```python
from build123d import *

# Parameters (mm, degrees)
SKETCH1_W               = 4
SKETCH1_H               = 2
SKETCH1_H_2             = 5
CUT_EXTRUDE1_DEPTH      = 94.386294498
CUT_EXTRUDE1_DEPTH_BACK = 94.386294498
SKETCH2_R               = 11


with BuildPart() as part:
    # Sketch1 → Revolve1 (revolve)
    with BuildSketch(Plane.YZ, mode=Mode.PRIVATE) as revolve1_sk:
        with BuildLine():
            ThreePointArc((-46, 2), (-23.174880185, 6.257119382), (0, 7.683334091))
            Line((0, 7.683334091), (0, 2))
            Line((0, 2), (-46, 2))
        make_face()
        Polygon((-46, 2), (-46, 0), (-42, 0), (0, 0), (0, 2), align=None)
        Polygon((0, 0), (-42, 0), (-42, -3), (-42, -5), (-42, -8), (-42, -10), (-42, -13), (-42, -15), (-42, -18), (-42, -20), (-42, -57), (-42, -59), (-42, -62), (-42, -67), (-37, -67), (-37, -58), (-25, -58), (-25, -22), (-37, -22), (-37, -5), (0, -5), align=None)
        with Locations((-44, -4)):
            Rectangle(SKETCH1_W, SKETCH1_H)
        with Locations((-44, -9)):
            Rectangle(SKETCH1_W, SKETCH1_H)
        with Locations((-44, -19)):
            Rectangle(SKETCH1_W, SKETCH1_H)
        with Locations((-44, -14)):
            Rectangle(SKETCH1_W, SKETCH1_H)
        with Locations((-44, -58)):
            Rectangle(SKETCH1_W, SKETCH1_H)
        with Locations((-44, -64.5)):
            Rectangle(SKETCH1_W, SKETCH1_H_2)
    revolve(revolve1_sk.sketch.rotate(Axis((0, 0, 0), (0, 0, 1)), 270), axis=Axis((0, 0, 0), (0, 0, 1)))

    # Sketch2 → Cut-Extrude1 (cut, two sides: drawn at the far end of the back side and taken through both)
    with BuildSketch(Plane(origin=(0, 0, 0), x_dir=(-1, 0, 0), z_dir=(0, 1, 0)).offset(-CUT_EXTRUDE1_DEPTH_BACK)):
        with Locations(Location((0, -40, 0), (0, 0, 90))):
            Circle(SKETCH2_R)
    extrude(amount=CUT_EXTRUDE1_DEPTH + CUT_EXTRUDE1_DEPTH_BACK, mode=Mode.SUBTRACT)


solid = part.part
```
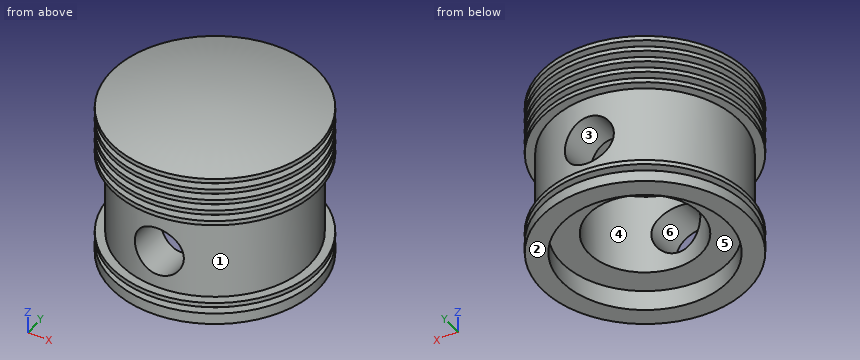
Model file for the job. Use its own axes, mm. Face numbers are marked on the shaded views. A direction names the side the tool comes from. Coordinates: 2 decimals unless noted, no trailing zeros. Loops run counter-clockwise (first coordinate to the right, second up) from the corner with the lowest first, then second, coordinate; pieces in that order, holes last. Notation, with made-up numbers: (-22.75, 70) - (29.25, 70) arc R33 ccw to (29.25, 105) - close; hole circle Ø10 at (21, 16.25). An arc over 180 degrees is marked (long way). Write item = value, one per line. Start each with the question number.
Item 1: Saw through at A-A, the plane z = -40. List the corners of the cut face in (x, y), then the cut area to 3 significant figures.
Item 2: Saw through at B-B, the plane x = 0. State how many separate pieces and enclosed holes the cut face has, then the cut area to 3 significant figures.
Item 3: Drop flat-ended pins along their axis: pin 1 Ø5 at (y, z) = (-10, -10.5) entering from -X; pin 2 Ø1 at (y, z) = (15, -36.5) entering from +X; pin 3 Ø3 at (x, z) = (33, -57) entering from +Y. Give the stop position or say it passes through.
Item 4: 3-axis set-ups, long thin cutter, end or side, ignore diameter. For the marked faces 5 and 6: which of +Z, -Z, +X, -X, +Y, -Y reach the whole face in a straight line?
Item 5: Pull direction X, two halves, no side cores. Call the marked faces 1, 2, 3 and 4: +X half, -X half, draft (parallel to the pull), parting line (faces both ways), or undercut.
Item 6: Wall check: probe 1 along Y at (x, z) = (0, -9); probe 2 along Z at (x, y) = (0, -34); probe 3 along Z at (x, y) = (0, -33.5). Give the ranges that are in metal, low to high. Write a range as [from, to].
Answers:
q1.outline = (-11, -40.53) - (-11, -22.45) arc R25 cw to (-11, 22.45) - (-11, 40.53) arc R42 ccw to start; (11, -40.53) arc R42 ccw to (11, 40.53) - (11, 22.45) arc R25 cw to (11, -22.45) - close
q1.area = 2,820 mm2
q2.separate_pieces = 3
q2.enclosed_holes = 0
q2.area = 1,810 mm2
q3.pin_1 = -45.38
q3.pin_2 = 39.42
q3.pin_3 = 33.52
q4.face_5 = -Z
q4.face_6 = +Y, -Y
q5.face_1 = parting line
q5.face_2 = draft
q5.face_3 = undercut
q5.face_4 = undercut
q6.probe_1 = [-46, -37], [37, 46]
q6.probe_2 = [-58, -51], [-29, -22], [-5, 4.6]
q6.probe_3 = [-58, -51], [-29, -22], [-5, 4.69]
